```python
from build123d import *

# Parameters (mm, degrees)
M3_TAPPED_HOLE1_D            = 2.5
M3_TAPPED_HOLE1_DEPTH        = 8
M3_TAPPED_HOLE1_TIP          = 0.751075774
F_3_0_3_DIAMETER_HOLE1_D     = 3
F_3_0_3_DIAMETER_HOLE1_DEPTH = 3
F_3_0_3_DIAMETER_HOLE1_TIP   = 0.901290929
M3_TAPPED_HOLE2_D            = 2.5
M3_TAPPED_HOLE2_DEPTH        = 12
M3_TAPPED_HOLE2_TIP          = 0.751075774
CHAMFER1_SIZE                = 0.5


with BuildPart() as part:
    # Sketch1 → Revolve1 (revolve)
    with BuildSketch(Plane.XY):
        Polygon((0, 0), (0, 3.5), (8.5, 3.5), (8.5, 7.5), (15, 7.5), (15, 0), align=None)
    revolve(axis=Axis((0, 0, 0), (1, 0, 0)))

    # M3 Tapped Hole1
    with Locations(Plane.ZY):
        with Locations((0, 0)):
            Hole(M3_TAPPED_HOLE1_D / 2, depth=M3_TAPPED_HOLE1_DEPTH)
            with Locations((0, 0, -(M3_TAPPED_HOLE1_DEPTH + M3_TAPPED_HOLE1_TIP / 2))):  # 118° drill point
                Cone(0, M3_TAPPED_HOLE1_D / 2, M3_TAPPED_HOLE1_TIP, mode=Mode.SUBTRACT)

    # Ø3.0 (3) Diameter Hole1
    with Locations(Plane(origin=(15, 0, 0), x_dir=(0, 0, -1), z_dir=(1, 0, 0))):
        with Locations((0, 0)):
            Hole(F_3_0_3_DIAMETER_HOLE1_D / 2, depth=F_3_0_3_DIAMETER_HOLE1_DEPTH)
            with Locations((0, 0, -(F_3_0_3_DIAMETER_HOLE1_DEPTH + F_3_0_3_DIAMETER_HOLE1_TIP / 2))):  # 118° drill point
                Cone(0, F_3_0_3_DIAMETER_HOLE1_D / 2, F_3_0_3_DIAMETER_HOLE1_TIP, mode=Mode.SUBTRACT)

    # M3 Tapped Hole2
    with Locations(Plane.XY.offset(7.5)):
        with Locations((11.75, 0)):
            Hole(M3_TAPPED_HOLE2_D / 2, depth=M3_TAPPED_HOLE2_DEPTH)
            with Locations((0, 0, -(M3_TAPPED_HOLE2_DEPTH + M3_TAPPED_HOLE2_TIP / 2))):  # 118° drill point
                Cone(0, M3_TAPPED_HOLE2_D / 2, M3_TAPPED_HOLE2_TIP, mode=Mode.SUBTRACT)

    # Chamfer1
    chamfer1_edges = [part.edges().sort_by_distance(p)[0] for p in [
        (15, -7.5, 0),
        (8.5, -7.5, 0),
        (0, -3.5, 0),
    ]]
    chamfer(chamfer1_edges, length=CHAMFER1_SIZE)


solid = part.part
```
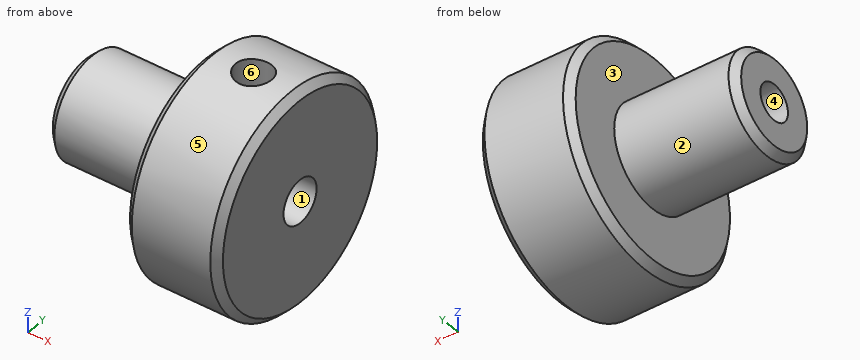
For this review, take the finished solid that the model builds, in its own axes (mm). Face numbers are marked on the shaded views. A direction names the side the tool comes from. Round coordinates to 2 decimals unless told otherwise and drop trailing zeros. Order: outer loops, then holes, each group sorted by start corner. A loop starts at its lowest first (then second) coordinate and runs counter-clockwise, first axis right, second up.
Q1. Machinability: for the marked faces 5 and 6, which of the approach directions +Z, -Z, +X, -X, +Y, -Y give a long, thin tool a straight path to every point of the face, cutting with its end or side? Answer none if there is none.
Findings below:
face 5: +X, -X
face 6: +Z
Q2. We need section C-C, the plane x = 13.25. Give the boundary of the cut face in (y, z), plus the area to 3 significant figures.
Findings below:
outline: circle Ø15 at (0, 0); hole circle Ø3 at (0, 0)
area: 170 mm2
Q3. We need section B-B, the plane x = 9.25. Give the boundary of the cut face in (y, z), plus the area to 3 significant figures.
Findings below:
outline: circle Ø15 at (0, 0)
area: 177 mm2
Q4. Mouldability with a two-part tool opening along Y and no side actions: class the marked faces 1, 2, 3 and 4 as pulls with the +Y half, pulls with the -Y half, needs draft (parallel to the pull), parting line crosses it, or undercut.
Findings below:
face 1: undercut
face 2: parting line crosses it
face 3: needs draft
face 4: undercut
Q5. Wall thickness on line 1 (Z direction, x = 14.25, y = 0); line 2 (Z direction, x = 3.25, y = 0); line 3 (X direction, y = 0, z = 4.5): over which ranges is each line inside the solid? List them lowest first.
Findings below:
line 1: z = -7.5 to -1.5, 1.5 to 7.5
line 2: z = -3.5 to -1.25, 1.25 to 3.5
line 3: x = 8.5 to 10.5, 13 to 15
Q6. We need section A-A, the plane x = 2.75. Give the boundary of the cut face in (y, z).
Findings below:
outline: circle Ø7 at (0, 0); hole circle Ø2.5 at (0, 0)
Q7. Insertion check: P1, Ø2, axis at y = 0, z = 0, coming from the -X side; P2, Ø4, axis at y = -6, z = -5, coming from the -X side; P3, Ø4, axis at y = 2.5, z = 4.5, coming from the -X side. Each pin has a flat end and moves straight along its axis. Give the tip position at first contact, or say it passes through.
Findings below:
P1: stops at x = 8.15
P2: stops at x = 8.5
P3: stops at x = 0.15
